Verification items for the finished model (mm, model axes). Coordinates: 2 decimals unless noted, no trailing zeros. Write each loop counter-clockwise with the first axis right and the second up, starting at its lowest first coordinate (ties: lowest second). Pieces come first, ordered by that corner, then holes. Notation, with made-up numbers: (-1, 71) -> (28, 71) arc R18 ccw to (28, 77) -> close; hole circle Ø9 at (-36.75, -17.75). An arc over 180 degrees is marked (long way). Use CSV: the item, a comma, the result in double quotes.
Autodesk Inventor part; units mm, degrees
ref_plane "YZ Plane" through (0, 0, 0) normal (1, 0, 0) x (0, 1, 0)
ref_plane "XZ Plane" through (0, 0, 0) normal (0, 1, 0) x (-1, 0, 0)
ref_plane "XY Plane" through (0, 0, 0) normal (0, 0, 1) x (1, 0, 0)
sketch "Sketch1" plane through (0, 0, 0) normal (0, 0, 1) x (1, 0, 0)
  line L0 (-67.4611, 97.9784) -> (62.5389, 97.9784)
  line L1 (62.5389, 97.9784) -> (62.5389, -175.0216)
  line L2 (62.5389, -175.0216) -> (-67.4611, -175.0216)
  line L3 (-67.4611, -175.0216) -> (-67.4611, 97.9784)
  circle A0 centre (-2.4611, -38.5216) radius 19.05
  line L4 (-67.4611, -38.5216) -> (62.5389, -38.5216) construction
  line L5 (-2.4611, 97.9784) -> (-2.4611, -175.0216) construction
  point P0 (0, 0)
  point P1 (-2.4611, -38.5216)
  dimension "d0" = 38.1
  dimension "d3" = 130
  dimension "d4" = 273
extrude "Extrusion1" add sketch "Sketch1" along normal blind 12.7
sketch "Sketch2" plane through (0, 0, 0) normal (0, 0, -1) x (-1, 0, 0)
  line L0 (67.4611, -175.0216) -> (-62.5389, -175.0216)
  line L1 (67.4611, 97.9784) -> (67.4611, -175.0216)
  line L2 (-62.5389, 97.9784) -> (67.4611, 97.9784)
  line L3 (-62.5389, -175.0216) -> (-62.5389, 97.9784)
  circle A0 centre (2.4611, -38.5216) radius 19.05
  line L4 (2.4611, -38.5216) -> (2.4611, -25.0418)
  line L5 (2.4611, -25.0418) -> (2.4611, -38.5216)
  line L6 (14.6161, -38.5216) -> (2.4611, -38.5216)
  point P0 (0, 0)
  point P1 (42.4611, 76.4784)
  point P2 (-37.5389, 76.4784)
  point P3 (-37.5389, -153.5216)
  point P4 (42.4611, -153.5216)
  dimension "d5" = 230
  dimension "d6" = 80
  dimension "d7" = 80
  dimension "d8" = 230
hole "Hole1" at (-42.4611, 76.4784, 0) at (37.5389, 76.4784, 0) at (37.5389, -153.5216, 0) at (-42.4611, -153.5216, 0) direction (0, 0, 1) diameter 12 end through all
properties part number "placa superior"
1) Cross-section at A-A (x = -4). Record the boundary of the cut face in (y, z).
Return value:
outline,"(-175.02, 0) -> (-57.51, 0) -> (-57.51, 12.7) -> (-175.02, 12.7) -> close; (-19.53, 0) -> (97.98, 0) -> (97.98, 12.7) -> (-19.53, 12.7) -> close"
2) Mould release check, pull along X, two halves, no side actions. Record for faces 1 (the cylindrical face through (-16.5, -51.4, 6.3)), 2 (the flat face through (62.539, -37, 6)), 3 (the flat face through (-2, -175.022, 6)): released by +X, released by -X, zero draft, split by the parting line, or undercut.
Return value:
face 1,"undercut"
face 2,"released by +X"
face 3,"zero draft"
3) Cross-section at B-B (y = -49). Record the boundary of the cut face in (x, z).
Return value:
outline,"(-67.46, 0) -> (-18.37, 0) -> (-18.37, 12.7) -> (-67.46, 12.7) -> close; (13.45, 0) -> (62.54, 0) -> (62.54, 12.7) -> (13.45, 12.7) -> close"
4) Cross-section at D-D (z = 2.75). Record the boundary of the cut face in (x, y).
Return value:
outline,"(-67.46, -175.02) -> (62.54, -175.02) -> (62.54, 97.98) -> (-67.46, 97.98) -> close; hole circle Ø12 at (-42.46, -153.52); hole circle Ø12 at (-42.46, 76.48); hole circle Ø38.1 at (-2.46, -38.52); hole circle Ø12 at (37.54, -153.52); hole circle Ø12 at (37.54, 76.48)"
5) Cross-section at C-C (x = 40). Record the boundary of the cut face in (y, z), plus the area to 3 significant figures.
Return value:
outline,"(-175.02, 0) -> (-158.99, 0) -> (-158.99, 12.7) -> (-175.02, 12.7) -> close; (-148.05, 0) -> (71.01, 0) -> (71.01, 12.7) -> (-148.05, 12.7) -> close; (81.95, 0) -> (97.98, 0) -> (97.98, 12.7) -> (81.95, 12.7) -> close"
area,"3,190 mm2"
6) Scan lines: L1, parallel to X at y = 81, z = 11.75; L2, parallel to Y at x = -2.5, z = 5.25; L3, parallel to X at y = 78, z = 9.5. Record each from-to range of solid material in increasing order.
Return value:
L1,"-67.46 to -46.41, -38.52 to 33.59, 41.48 to 62.54"
L2,"-175.02 to -57.57, -19.47 to 97.98"
L3,"-67.46 to -48.26, -36.66 to 31.74, 43.34 to 62.54"
